Geometry check sheet. Reference: the model listing, model coordinates, mm. Face numbers are marked on the shaded views. A direction names the side the tool comes from. Give positions to 0.01 mm unless a question says otherwise; leave off trailing zeros. Loops run counter-clockwise (first coordinate to the right, second up) from the corner with the lowest first, then second, coordinate; pieces in that order, holes last.
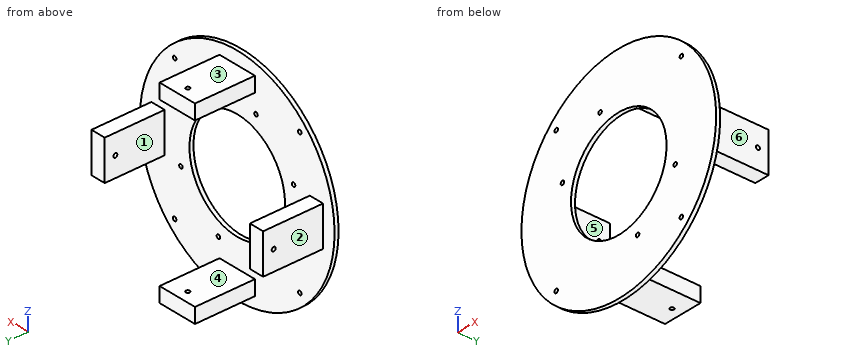
Autodesk Fusion 360 part; units mm, degrees
sketch "Sketch1" plane through (0, 0, 0) normal (0, 1, 0) x (1, 0, 0)
  circle A0 centre (0, 0) radius 27
  circle A1 centre (0, 0) radius 55
  line L0 (10, -41) -> (-10, -41)
  line L1 (-10, -41) -> (-10, -48.5)
  line L2 (-10, -48.5) -> (10, -48.5)
  line L3 (10, -48.5) -> (10, -41)
  line L4 (10, -41) -> (-10, -48.5) construction
  line L5 (-10, -41) -> (10, -48.5) construction
  line L6 (41, 10) -> (48.5, -10) construction
  line L7 (41, 10) -> (41, -10)
  line L8 (48.5, -10) -> (48.5, 10)
  line L9 (48.5, 10) -> (41, 10)
  line L10 (41, -10) -> (48.5, 10) construction
  line L11 (41, -10) -> (48.5, -10)
  line L12 (-10, 41) -> (10, 48.5) construction
  line L13 (-10, 41) -> (10, 41)
  line L14 (10, 48.5) -> (-10, 48.5)
  line L15 (-10, 48.5) -> (-10, 41)
  line L16 (10, 41) -> (-10, 48.5) construction
  line L17 (10, 41) -> (10, 48.5)
  line L18 (-41, -10) -> (-48.5, 10) construction
  line L19 (-41, -10) -> (-41, 10)
  line L20 (-48.5, 10) -> (-48.5, -10)
  line L21 (-48.5, -10) -> (-41, -10)
  line L22 (-41, 10) -> (-48.5, -10) construction
  line L23 (-41, 10) -> (-48.5, 10)
  line L24 (0, 0) -> (0, -44.75)
  line L25 (0, 0) -> (27, 0)
  point P0 (0, -44.75)
  point P1 (44.75, 0)
  point P2 (0, 44.75)
  point P3 (-44.75, 0)
  dimension "d1" = 54
  dimension "d2" = 110
  dimension "d7" = 7.5
  dimension "d8" = 20
  dimension "d9" = 41
  dimension "d11" = 360
extrude "Extrude3" add sketch "Sketch1" along normal blind 2 contours L0 L1 L2 L3 | A1 | L7 L8 L9 L11 | L13 L14 L15 L17 | L19 L20 L21 L23
extrude "Extrude5" add sketch "Sketch1" along normal blind 32 contours L0 L1 L2 L3 | L7 L8 L9 L11 | L13 L14 L15 L17 | L19 L20 L21 L23
sketch "Sketch6" plane through (0, 2, 0) normal (0, 1, 0) x (-1, 0, 0)
  line L0 (-10, 48.5) -> (10, 48.5)
  line L1 (10, 48.5) -> (10, 41)
  line L2 (10, 41) -> (-10, 41)
  line L3 (-10, 41) -> (-10, 48.5)
  line L4 (41, -10) -> (41, 10)
  line L5 (41, 10) -> (48.5, 10)
  line L6 (48.5, 10) -> (48.5, -10)
  line L7 (48.5, -10) -> (41, -10)
  line L8 (-41, 10) -> (-41, -10)
  line L9 (-41, -10) -> (-48.5, -10)
  line L10 (-48.5, -10) -> (-48.5, 10)
  line L11 (-48.5, 10) -> (-41, 10)
  line L12 (-10, -41) -> (10, -41)
  line L13 (10, -41) -> (10, -48.5)
  line L14 (10, -48.5) -> (-10, -48.5)
  line L15 (-10, -48.5) -> (-10, -41)
  circle A0 centre (0, 0) radius 27
  circle A1 centre (0, 0) radius 55
  line L16 (29.6985, 15.5563) -> (26.8701, 12.7279)
  line L17 (12.7279, 26.8701) -> (15.5563, 29.6985)
  line L18 (18.1297, 22.7228) -> (20.9915, 22.7228) construction
  line L19 (15.3614, 25.1762) -> (18.4198, 25.1762) construction
  line L20 (17.8019, 25.9553) -> (17.4822, 25.9553) construction
  line L21 (29.6985, 15.5563) -> (26.8701, 12.7279)
  line L22 (26.8701, 12.7279) -> (22.6274, 16.9706)
  line L23 (22.6274, 16.9706) -> (25.4558, 19.799)
  line L24 (25.4558, 19.799) -> (29.6985, 15.5563)
  line L25 (15.5563, 29.6985) -> (12.7279, 26.8701)
  line L26 (12.7279, 26.8701) -> (16.9706, 22.6274)
  line L27 (16.9706, 22.6274) -> (19.799, 25.4558)
  line L28 (19.799, 25.4558) -> (15.5563, 29.6985)
  line L29 (22.6274, 16.9706) -> (16.9706, 22.6274)
  line L30 (0, 0) -> (27, 0)
  line L31 (0, 0) -> (19.799, 19.799)
  line L32 (-15.3614, -25.1762) -> (-18.4198, -25.1762) construction
  line L33 (-22.6274, -16.9706) -> (-25.4558, -19.799)
  line L34 (-12.7279, -26.8701) -> (-15.5563, -29.6985)
  line L35 (-26.8701, -12.7279) -> (-22.6274, -16.9706)
  line L36 (-12.7279, -26.8701) -> (-16.9706, -22.6274)
  line L37 (-25.4558, -19.799) -> (-29.6985, -15.5563)
  line L38 (-29.6985, -15.5563) -> (-26.8701, -12.7279)
  line L39 (-18.1297, -22.7228) -> (-20.9915, -22.7228) construction
  line L40 (-29.6985, -15.5563) -> (-26.8701, -12.7279)
  line L41 (-19.799, -25.4558) -> (-15.5563, -29.6985)
  line L42 (-16.9706, -22.6274) -> (-19.799, -25.4558)
  line L43 (-22.6274, -16.9706) -> (-16.9706, -22.6274)
  line L44 (-15.5563, -29.6985) -> (-12.7279, -26.8701)
  line L45 (-17.8019, -25.9553) -> (-17.4822, -25.9553) construction
  circle A2 centre (35.3553, -35.3553) radius 1
  line L46 (35.3553, -35.3553) -> (0, 0)
  circle A3 centre (35.3553, 35.3553) radius 1
  circle A4 centre (-35.3553, 35.3553) radius 1
  circle A5 centre (-35.3553, -35.3553) radius 1
  circle A6 centre (31.8198, 10.6066) radius 1
  line L47 (28.2843, 14.1421) -> (31.8198, 10.6066)
  line L48 (19.799, 19.799) -> (22.225, 22.225)
  circle A7 centre (10.6066, 31.8198) radius 1
  circle A8 centre (-31.8198, -10.6066) radius 1
  circle A9 centre (-10.6066, -31.8198) radius 1
  point P0 (19.799, 19.799)
  point P1 (-19.799, -19.799)
  point P2 (-19.799, -19.799)
  dimension "d37" = 4
  dimension "d38" = 20
  dimension "d43" = 6
  dimension "d44" = 6
  dimension "d45" = 4
  dimension "d46" = 45
  dimension "d48" = 360
  dimension "d61" = 2
  dimension "d62" = 45
  dimension "d63" = 50
  dimension "d65" = 360
  dimension "d68" = 2
  dimension "d69" = 5
  dimension "d71" = 360
  dimension "d74" = 16
  dimension "d75" = 28
extrude "Extrude12" cut sketch "Sketch6" against normal blind 30 contours A6 | A7 | A8 | A9
extrude "Extrude11" cut sketch "Sketch6" against normal blind 10 contours A2 | A3 | A4 | A5
sketch "Sketch8" plane through (0, 0, 48.5) normal (0, 0, 1) x (1, 0, 0)
  line L0 (-10, 2) -> (10, 2)
  line L1 (10, 2) -> (10, 32)
  line L2 (10, 32) -> (-10, 32)
  line L3 (-10, 32) -> (-10, 2)
  circle A0 centre (0, 26.7) radius 1
  dimension "d51" = 2
  dimension "d52" = 10
  dimension "d53" = 24.7
extrude "Extrude9" cut sketch "Sketch8" against normal blind 100 contours A0
sketch "Sketch9" plane through (48.5, 0, 0) normal (1, 0, 0) x (0, 0, -1)
  line L0 (-10, 2) -> (10, 2)
  line L1 (10, 2) -> (10, 32)
  line L2 (10, 32) -> (-10, 32)
  line L3 (-10, 32) -> (-10, 2)
  circle A0 centre (0, 26.7) radius 1
  dimension "d56" = 2
  dimension "d57" = 10
  dimension "d58" = 24.7
extrude "Extrude10" cut sketch "Sketch9" against normal blind 100 contours A0
sketch "Sketch10" plane through (0, 2, 0) normal (0, 1, 0) x (-1, 0, 0)
  circle A0 centre (35.3553, 35.3553) radius 1
  circle A1 centre (-35.3553, 35.3553) radius 1
  circle A2 centre (35.3553, -35.3553) radius 1
  circle A3 centre (-35.3553, -35.3553) radius 1
  circle A4 centre (-31.8198, -10.6066) radius 1
  circle A5 centre (31.8198, 10.6066) radius 1
  circle A6 centre (-10.6066, -31.8198) radius 1
  circle A7 centre (10.6066, 31.8198) radius 1
  line L0 (-10, 48.5) -> (10, 48.5)
  line L1 (10, 48.5) -> (10, 41)
  line L2 (10, 41) -> (-10, 41)
  line L3 (-10, 41) -> (-10, 48.5)
  line L4 (41, -10) -> (41, 10)
  line L5 (41, 10) -> (48.5, 10)
  line L6 (48.5, 10) -> (48.5, -10)
  line L7 (48.5, -10) -> (41, -10)
  line L8 (-41, 10) -> (-41, -10)
  line L9 (-41, -10) -> (-48.5, -10)
  line L10 (-48.5, -10) -> (-48.5, 10)
  line L11 (-48.5, 10) -> (-41, 10)
  line L12 (-10, -41) -> (10, -41)
  line L13 (10, -41) -> (10, -48.5)
  line L14 (10, -48.5) -> (-10, -48.5)
  line L15 (-10, -48.5) -> (-10, -41)
  circle A8 centre (0, 0) radius 27
  circle A9 centre (0, 0) radius 55
1) Mould release check, pull along X, two halves, no side actions. Record for the marked faces 4, 5 and 6: +X half, -X half, draft (parallel to the pull), parting line (faces both ways), or undercut.
2) Sectioned sample at D-D on x = -3. Enter the section's corners in (y, z).
3) Tool access check on the marked faces 1, 2 and 3. Record the directions out of +Z, -Z, +X, -X, +Y, -Y that give a thin tool (end or side, any length) a straight path to the whole face; none if there is none.
4) Sectioned sample at C-C on x = 19. Enter the section's corners in (y, z), plus the area to 3 significant figures.
5) Sectioned sample at B-B on z = 22.5. Enter the section's corners in (x, y), plus the area to 3 significant figures.
6) Depth check by flat-ended pin: P1, Ø6, axis at y = 22, z = -2, coming from the +X side; P2, Ø16, axis at x = -1.5, y = 15.5, coming from the -Z side; P3, Ø1.6, axis at x = -35.36, z = -35.36, coming from the +Y side; P4, Ø3, axis at y = 26.7, z = 0, coming from the -X side. Enter the tip coordinate at first touch or a pass-through.
7) Sectioned sample at A-A on y = 30. Enter the section's corners in (x, z).
8) Scan lines: line 1 along Z through (x, y) = (-5, 21); line 2 along Y through (x, z) = (-35.5, -20). Record each from-to range of solid material in increasing order.
Determined:
1. face 4: draft
1. face 5: undercut
1. face 6: +X half
2. outline: (0, -54.92) - (2, -54.92) - (2, -48.5) - (32, -48.5) - (32, -41) - (2, -41) - (2, -26.83) - (0, -26.83) - close; (0, 26.83) - (2, 26.83) - (2, 41) - (32, 41) - (32, 48.5) - (2, 48.5) - (2, 54.92) - (0, 54.92) - close
3. face 1: +Z, -Z, +Y
3. face 2: +Z, -Z, -X, +Y
3. face 3: +Z, +X, -X, +Y
4. outline: (0, -51.61) - (2, -51.61) - (2, -19.18) - (0, -19.18) - close; (0, 19.18) - (2, 19.18) - (2, 51.61) - (0, 51.61) - close
4. area: 130 mm2
5. outline: (-50.19, 0) - (-14.92, 0) - (-14.92, 2) - (-50.19, 2) - close; (14.92, 0) - (50.19, 0) - (50.19, 2) - (14.92, 2) - close
5. area: 141 mm2
6. P1: stops at x = 48.5
6. P2: stops at z = -48.5
6. P3: passes through
6. P4: stops at x = -48.5
7. outline: (-48.5, -10) - (-41, -10) - (-41, 10) - (-48.5, 10) - close; (-10, -48.5) - (10, -48.5) - (10, -41) - (-10, -41) - close; (-10, 41) - (10, 41) - (10, 48.5) - (-10, 48.5) - close; (41, -10) - (48.5, -10) - (48.5, 10) - (41, 10) - close
8. line 1: z = -48.5 to -41, 41 to 48.5
8. line 2: y = 0 to 2
